Build history of the part. All positions in model axes, mm. A direction names the side the tool comes from. Give positions to 0.01 mm unless a question says otherwise; leave off trailing zeros. Loops run counter-clockwise (first coordinate to the right, second up) from the corner with the lowest first, then second, coordinate; pieces in that order, holes last. Notation, with made-up numbers: (-23, 46) -> (8, 46) arc R9 ccw to (8, 63) -> close; hole circle Ø4 at (17.5, 16.25). An arc over 180 degrees is marked (long way). One line per question, with ' | ' between items. Start each with the question number.
(1) Slice it at D-D, the plane y = 11.5. Write the cut outline in (x, z).
(2) Drill centre lines: L1, parallel to Z at x = 0, y = -8; L2, parallel to X at y = -7, z = 0 (3 decimals); L3, parallel to Z at x = 0, y = -5. Where is each one in solid material? Low to high. Write a range as from..to.
(3) Mould opens along X. For faces 1 (the face through (5, 10, 0)), 2 (the face through (-2.5, -16, -2.5)) say: pulls with the +X half, pulls with the -X half, needs draft (parallel to the pull), parting line crosses it, or undercut.
(4) Slice it at A-A, the plane z = 0. Write the cut outline in (x, y).
(5) Slice it at B-B, the plane y = 6. Write the cut outline in (x, z), then the cut area to 3 significant figures.
(6) 3-axis set-ups, long thin cutter, end or side, ignore diameter. For faces 3 (the face through (2.2, 0, 2.5)), 4 (the face through (-3, -8, 0)): which of +Z, -Z, +X, -X, +Y, -Y reach the whole face in a straight line?
(7) Slice it at C-C, the plane x = -7. Write the cut outline in (y, z) (3 decimals), then the cut area to 3 significant figures.
(8) Flat gauge pins, fed straight in: pin 1 Ø3 at (y, z) = (9, 1) entering from -X; pin 2 Ø5 at (x, y) = (4.5, -11.5) entering from +Z; pin 3 Ø1.7 at (y, z) = (14.5, -0.5) entering from +X. Where does each tip first touch, or does it go through?
```python
from build123d import *

# Parameters (mm, degrees)
ENL_V_MAT_EXTRU_1_DEPTH      = 21
ESQUISSE3_R                  = 3
ENL_V_MAT_EXTRU_2_DEPTH      = 21
ENL_V_MAT_EXTRU_3_DEPTH      = 21
ENL_V_MAT_EXTRU_3_DEPTH_BACK = 21


with BuildPart() as part:
    # Esquisse1 → Révolution1 (revolve)
    with BuildSketch(Plane.XY):
        with BuildLine():
            Line((0, 20), (0, -20))
            ThreePointArc((0, -20), (20, 0), (0, 20))
        make_face()
    revolve(axis=Axis((0, 38.8303663, 0), (0, -1, 0)))

    # Esquisse2 → Enlèv. mat.-Extru.1 (cut, through all)
    with BuildSketch(Plane(origin=(0, 0, 0), x_dir=(1, 0, 0), z_dir=(0, 1, 0))):
        Polygon((5, -2.886751346), (5, 2.886751346), (0, 5.773502692), (-5, 2.886751346), (-5, -2.886751346), (0, -5.773502692), align=None)
    extrude(amount=ENL_V_MAT_EXTRU_1_DEPTH, mode=Mode.SUBTRACT)

    # Esquisse3 → Enlèv. mat.-Extru.2 (cut, through all)
    with BuildSketch(Plane(origin=(0, 0, 0), x_dir=(1, 0, 0), z_dir=(0, 1, 0))):
        Circle(ESQUISSE3_R)
    extrude(amount=-ENL_V_MAT_EXTRU_2_DEPTH, mode=Mode.SUBTRACT)

    # Esquisse5 → Enlèv. mat.-Extru.3 (cut, two sides)
    with BuildSketch(Plane.XY) as enl_v_mat_extru_3_sk:
        Polygon((188.012399008, -16), (31.726859594, -16), (-44.024896915, -16), (-200.310436329, -16), (-200.310436329, -328.571078828), (188.012399008, -328.571078828), align=None)
    extrude(amount=ENL_V_MAT_EXTRU_3_DEPTH, mode=Mode.SUBTRACT)
    extrude(enl_v_mat_extru_3_sk.sketch, amount=-ENL_V_MAT_EXTRU_3_DEPTH_BACK, mode=Mode.SUBTRACT)


solid = part.part
```
Final values:
1) outline: circle Ø32.73 at (0, 0); hole (-5, -2.89) -> (0, -5.77) -> (5, -2.89) -> (5, 2.89) -> (0, 5.77) -> (-5, 2.89) -> close
2) L1: -18.33..-3, 3..18.33 | L2: -18.735..-3, 3..18.735 | L3: -19.36..-3, 3..19.36
3) face 1: undercut | face 2: needs draft
4) outline: (-12, -16) -> (-3, -16) -> (-3, 0) -> (-5, 0) -> (-5, 19.36) arc R20 ccw to start; (3, -16) -> (12, -16) arc R20 ccw to (5, 19.36) -> (5, 0) -> (3, 0) -> close
5) outline: circle Ø38.16 at (0, 0); hole (-5, -2.89) -> (0, -5.77) -> (5, -2.89) -> (5, 2.89) -> (0, 5.77) -> (-5, 2.89) -> close | area: 1,060 mm2
6) face 3: +Y | face 4: +Y, -Y
7) outline: (-16, -9.747) arc R18.735 ccw (long way) to (-16, 9.747) -> close | area: 1,070 mm2
8) pin 1: x = -18.52 | pin 2: z = 17.41 | pin 3: x = 14.61
